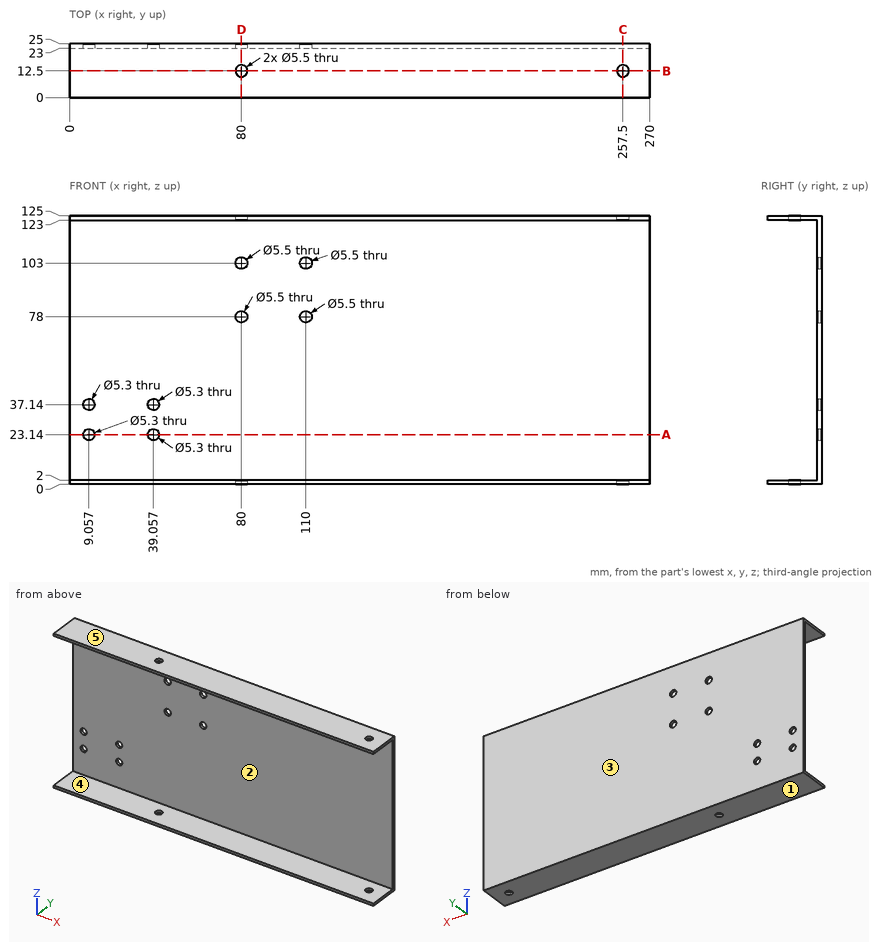
Geometry: see drawing. Coordinates: mm, zero at the bounding-box minimum. A direction names the side the tool comes from. Give positions to 0.01 mm unless a question says otherwise; leave off trailing zeros. Loops run counter-clockwise (first coordinate to the right, second up) from the corner with the lowest first, then second, coordinate; pieces in that order, holes last. Notation, with made-up numbers: M -17,82.5 L 38,82.5 A6 cw 38,87.5 Z; hole C -3,-22.5 d5. An arc over 180 degrees is marked long. Answer as CSV lines item,"result". Start each with the question number.
1. Pull-direction query (Z, two-part tool) for the marked faces 1, 2 and 3; classes: released by +Z, released by -Z, zero draft, split by the parting line, or undercut.
2. Section D-D on x = 80. Return loops of the section in (y, z), plus the area to 3 significant figures.
3. Section C-C on x = 257.5. Return loops of the section in (y, z).
4. Section A-A on z = 23.14. Return loops of the section in (x, y), plus the area to 3 significant figures.
5. Pin query (flat end, axial travel): P1, Ø2, axis at x = 116, z = 98, coming from the -Y side; P2, Ø4.5, axis at x = 80, y = 12.5, coming from the +Z side. Return the tip coordinate at first contact, or that it passes through.
6. Section B-B on y = 12.5. Return loops of the section in (x, z), plus the area to 3 significant figures.
7. Line query: L1, parallel to X at y = 23.85, z = 78; L2, parallel to X at y = 24.45, z = 37.14; L3, parallel to Z at x = 80, y = 23.5. Output: solid intervals per line, ascending.
8. Reachability of the marked faces 4 and 5 from +Z, -Z, +X, -X, +Y, -Y: full face, straight path, thin tool, end or side. Return the list, or none.
Computed values:
1,face 1,"released by -Z"
1,face 2,"undercut"
1,face 3,"zero draft"
2,outline,"M 0,0 L 9.75,0 L 9.75,2 L 0,2 Z; M 0,123 L 9.75,123 L 9.75,125 L 0,125 Z; M 15.25,0 L 25,0 L 25,75.25 L 23,75.25 L 23,2 L 15.25,2 Z; M 15.25,123 L 23,123 L 23,105.75 L 25,105.75 L 25,125 L 15.25,125 Z; M 23,80.75 L 25,80.75 L 25,100.25 L 23,100.25 Z"
2,area,"298 mm²"
3,outline,"M 0,0 L 9.75,0 L 9.75,2 L 0,2 Z; M 0,123 L 9.75,123 L 9.75,125 L 0,125 Z; M 15.25,0 L 25,0 L 25,125 L 15.25,125 L 15.25,123 L 23,123 L 23,2 L 15.25,2 Z"
4,outline,"M 0,23 L 6.41,23 L 6.41,25 L 0,25 Z; M 11.71,23 L 36.41,23 L 36.41,25 L 11.71,25 Z; M 41.71,23 L 270,23 L 270,25 L 41.71,25 Z"
4,area,"519 mm²"
5,P1,"stops at y = 23"
5,P2,"passes through"
6,outline,"M 0,0 L 77.25,0 L 77.25,2 L 0,2 Z; M 0,123 L 77.25,123 L 77.25,125 L 0,125 Z; M 82.75,0 L 254.75,0 L 254.75,2 L 82.75,2 Z; M 82.75,123 L 254.75,123 L 254.75,125 L 82.75,125 Z; M 260.25,0 L 270,0 L 270,2 L 260.25,2 Z; M 260.25,123 L 270,123 L 270,125 L 260.25,125 Z"
6,area,"1,040 mm²"
7,L1,"x = 0 to 77.25, 82.75 to 107.25, 112.75 to 270"
7,L2,"x = 0 to 6.41, 11.71 to 36.41, 41.71 to 270"
7,L3,"z = 0 to 75.25, 80.75 to 100.25, 105.75 to 125"
8,face 4,"+X, -X, -Y"
8,face 5,"+Z, +X, -X, +Y, -Y"
